Read the model definition and answer for the solid it produces. Units are mm, in the model's axes. A direction names the side the tool comes from. Coordinates: 2 decimals unless noted, no trailing zeros. Write each loop counter-clockwise with the first axis right and the second up, starting at its lowest first coordinate (ties: lowest second). Pieces come first, ordered by that corner, then holes.
1) Determine the mould class of faces 5 (the face through (10, 8, 0)), 6 (the face through (18.44, -17.48, 9.1)), 7 (the face through (-13.64, -17.48, -0.37)), 8 (the face through (0, -19, 0)) for opening direction Z: +Z half, -Z half, draft (parallel to the pull), parting line (faces both ways), or undercut.
2) The part is cut by section D-D (x = 0). Determine the outline of the cut face in (y, z), then the cut area to 3 significant figures.
3) Which of the six approach directions +Z, -Z, +X, -X, +Y, -Y give full straight-line access (tool end or side, diameter ignored) to faces 1 (the face through (10, -1, -8)), 2 (the face through (13, -16, 0)), 3 (the face through (7.9, -10, 9)), 4 (the face through (0, -6, -8))?
4) Find the intervals of material crossed by line 1 (X direction, y = -16.95, z = 0); line 2 (Z direction, x = 0, y = -16.8); line 3 (X direction, y = -9.5, z = -3), in increasing order.
5) Each of these flat-tipped pins is pushed along its axis until it touches: pin 1 Ø5.5 at (x, z) = (15.3, 0) entering from +Y; pin 2 Ø5 at (x, y) = (-9.5, 1) entering from -Z; pin 3 Ø3 at (x, z) = (0, 7.5) entering from +Y; pin 4 Ø3 at (y, z) = (-12, -5.318) entering from +X. Where does it stop, or does it pass through?
6) The part is cut by section C-C (y = -15). Determine the outline of the cut face in (x, z).
7) The part is cut by section A-A (x = -15.3). Determine the outline of the cut face in (y, z), then the cut area to 3 significant figures.
8) The part is cut by section B-B (z = 0). Determine the outline of the cut face in (x, y).
from build123d import *

# Parameters (mm, degrees)
ESQUISSE2_W                    = 2.5
ESQUISSE2_H                    = 6
BOSS_EXTRU_1_START             = -2.5
ESQUISSE3_R                    = 2
BOSS_EXTRU_1_DEPTH             = 2.5
BOSS_EXTRU_2_START             = -2.5
ESQUISSE3_3_W                  = 20
ESQUISSE3_3_H                  = 3
ESQUISSE3_3_W_2                = 2
BOSS_EXTRU_2_DEPTH             = 8.8
ESQUISSE3_5_W                  = 20
ESQUISSE3_5_H                  = 3
BOSS_EXTRUDE1_DEPTH            = 8
CUT_EXTRUDE1_REACH             = 34.38
SKETCH4_R                      = 1.7
TROUS_DE_CENTRAGE_2_0MM1_D     = 2
TROUS_DE_CENTRAGE_2_0MM1_DEPTH = 3
FILLET1_R                      = 1
FILLET2_START                  = -8.8
FILLET2_DEPTH                  = 17.6
FILLET2_START_2                = -19.3
FILLET2_2_DEPTH                = 38.6
FILLET3_R                      = 3


with BuildPart() as part:
    # Esquisse2 → Révolution1 (revolve)
    with BuildSketch(Plane.XY, mode=Mode.PRIVATE) as r_volution1_sk:
        with Locations((10.05, 5)):
            Rectangle(ESQUISSE2_W, ESQUISSE2_H)
    revolve(r_volution1_sk.sketch.rotate(Axis((-2.14668318, 0, 0), (1, 0, 0)), 90), axis=Axis((-2.14668318, 0, 0), (1, 0, 0)))

    # Esquisse3 → Boss.-Extru.1 (add)
    with BuildSketch(Plane(origin=(11.3, 0, 0), x_dir=(0, 0, -1), z_dir=(1, 0, 0)).offset(BOSS_EXTRU_1_START)):
        with BuildLine():
            Line((-10, -19), (10, -19))
            Line((10, -19), (10, -3.313708499))
            Line((10, -3.313708499), (8, -3.313708499))
            Line((8, -3.313708499), (8, 0))
            ThreePointArc((8, 0), (0, -8), (-8, 0))
            Line((-8, 0), (-8, -6.142135624))
            Line((-8, -6.142135624), (-10, -6.142135624))
            Line((-10, -6.142135624), (-10, -19))
        make_face()
        with Locations((5.318, -12)):
            Circle(ESQUISSE3_R, mode=Mode.SUBTRACT)
    extrude(amount=BOSS_EXTRU_1_DEPTH)

    # Esquisse3<3> → Boss.-Extru.2 (add)
    with BuildSketch(Plane(origin=(11.3, 0, 0), x_dir=(0, 0, -1), z_dir=(1, 0, 0)).offset(BOSS_EXTRU_2_START)):
        with Locations((0, -17.5)):
            Rectangle(ESQUISSE3_3_W, ESQUISSE3_3_H)
        with Locations((-9, -7.642135624)):
            Rectangle(ESQUISSE3_3_W_2, ESQUISSE3_3_H)
        with Locations((9, -4.813708499)):
            Rectangle(ESQUISSE3_3_W_2, ESQUISSE3_3_H)
    extrude(amount=-BOSS_EXTRU_2_DEPTH)

    # Esquisse3<5> → Boss-Extrude1 (add)
    with BuildSketch(Plane(origin=(11.3, 0, 0), x_dir=(0, 0, -1), z_dir=(1, 0, 0))):
        with Locations((0, -17.5)):
            Rectangle(ESQUISSE3_5_W, ESQUISSE3_5_H)
    extrude(amount=BOSS_EXTRUDE1_DEPTH)

    # Sketch4 → Cut-Extrude1 (cut, up to next)
    with BuildSketch(Plane(origin=(0, -16, 0), x_dir=(1, 0, 0), z_dir=(0, 1, 0)), mode=Mode.PRIVATE) as cut_extrude1_sk1:
        with Locations(Location((15.3, 0, 0), (0, 0, 270))):
            Circle(SKETCH4_R)
    cut_extrude1_tool1 = extrude(cut_extrude1_sk1.sketch, amount=-CUT_EXTRUDE1_REACH, mode=Mode.PRIVATE) & part.part
    add(cut_extrude1_tool1.solids().sort_by_distance((15.3, -16, 0))[0], mode=Mode.SUBTRACT)

    # Symétrie1: part across plane


with BuildPart() as part_1:
    add(part.part)
    add(part.part.mirror(Plane(origin=(0, 0, 0), x_dir=(0, 0, 1), z_dir=(1, 0, 0))))

    # Trous de centrage Ø2.0mm1
    with Locations(Plane(origin=(0, -16, 0), x_dir=(1, 0, 0), z_dir=(0, 1, 0))):
        with Locations((0, -7.5)):
            Hole(TROUS_DE_CENTRAGE_2_0MM1_D / 2, depth=TROUS_DE_CENTRAGE_2_0MM1_DEPTH)

    # Fillet1
    fillet1_edges = [part_1.edges().sort_by_distance(p)[0] for p in [
        (-10.05, -3.313708499, -8),
        (-10.05, -6.142135624, 8),
        (10.05, -3.313708499, -8),
        (10.05, -6.142135624, 8),
    ]]
    fillet(fillet1_edges, radius=FILLET1_R)

    # Fillet2: read off the stored shape, not the designer's step
    # Fillet2 outline → Fillet2 (cut)
    with BuildSketch(Plane.YZ.offset(FILLET2_START)):
        with BuildLine():
            ThreePointArc((-4.313708499, -8), (-3.606601718, -8.292893219), (-3.313708499, -9))
            Line((-3.313708499, -9), (-3.313708499, -8))
            Line((-3.313708499, -8), (-4.313708499, -8))
        make_face()
        with BuildLine():
            ThreePointArc((-3.313708499, -9), (-3.606601718, -9.707106781), (-4.313708499, -10))
            Line((-4.313708499, -10), (-3.313708499, -10))
            Line((-3.313708499, -10), (-3.313708499, -9))
        make_face()
        with BuildLine():
            Line((-6.142135624, 8), (-6.142135624, 9))
            ThreePointArc((-6.142135624, 9), (-6.435028843, 8.292893219), (-7.142135624, 8))
            Line((-7.142135624, 8), (-6.142135624, 8))
        make_face()
        with BuildLine():
            ThreePointArc((-7.142135624, 10), (-6.435028843, 9.707106781), (-6.142135624, 9))
            Line((-6.142135624, 9), (-6.142135624, 10))
            Line((-6.142135624, 10), (-7.142135624, 10))
        make_face()
    extrude(amount=FILLET2_DEPTH, mode=Mode.SUBTRACT)

    # Fillet2 2 outline → Fillet2 2 (cut)
    with BuildSketch(Plane.YZ.offset(FILLET2_START_2)):
        with BuildLine():
            ThreePointArc((-3.313708499, -9), (-3.606601718, -9.707106781), (-4.313708499, -10))
            Line((-4.313708499, -10), (-3.313708499, -10))
            Line((-3.313708499, -10), (-3.313708499, -9))
        make_face()
        with BuildLine():
            ThreePointArc((-7.142135624, 10), (-6.435028843, 9.707106781), (-6.142135624, 9))
            Line((-6.142135624, 9), (-6.142135624, 10))
            Line((-6.142135624, 10), (-7.142135624, 10))
        make_face()
    extrude(amount=FILLET2_2_DEPTH, mode=Mode.SUBTRACT)

    # Fillet3
    fillet3_edges = [part_1.edges().sort_by_distance(p)[0] for p in [
        (-8.8, -6.313708499, -9),
        (-19.3, -17.5, -10),
        (8.8, -6.313708499, -9),
        (8.8, -9.142135624, 9),
        (19.3, -17.5, -10),
        (19.3, -17.5, 10),
        (-8.8, -9.142135624, 9),
        (-19.3, -17.5, 10),
    ]]
    fillet(fillet3_edges, radius=FILLET3_R)


solid = part_1.part
Reported:
1. face 5: parting line
1. face 6: +Z half
1. face 7: undercut
1. face 8: draft
2. outline: (-19, -10) - (-16, -10) - (-16, 6.5) - (-19, 6.5) - close; (-19, 8.5) - (-16, 8.5) - (-16, 10) - (-19, 10) - close; (-9.14, 8) - (-7.14, 8) arc R1 ccw to (-7.14, 10) - (-9.14, 10) - close; (-6.31, -10) - (-4.31, -10) arc R1 ccw to (-4.31, -8) - (-6.31, -8) - close
2. area: 65.1 mm2
3. face 1: -Z, +X, -X, +Y
3. face 2: +Z, -Z, +X, +Y
3. face 3: +Z, -Z
3. face 4: +Y
4. line 1: x = -19.3 to -17, -13.6 to 13.6, 17 to 19.3
4. line 2: z = -10 to 6.5, 8.5 to 10
4. line 3: x = -11.3 to -8.8, 8.8 to 11.3
5. pin 1: stops at y = -16
5. pin 2: stops at z = -8
5. pin 3: stops at y = -6.14
5. pin 4: passes through
6. outline: (-11.3, -10) - (-8.8, -10) - (-8.8, 10) - (-11.3, 10) - close; (8.8, -10) - (11.3, -10) - (11.3, 10) - (8.8, 10) - close
7. outline: (-19, -10) - (-16, -10) - (-16, -1.7) - (-19, -1.7) - close; (-19, 1.7) - (-16, 1.7) - (-16, 10) - (-19, 10) - close
7. area: 49.8 mm2
8. outline: (-19.3, -19) - (-17, -19) - (-17, -16) - (-19.3, -16) - close; (-13.6, -19) - (13.6, -19) - (13.6, -16) - (11.3, -16) - (11.3, -2) - (8.8, -2) - (8.8, -16) - (-8.8, -16) - (-8.8, -2) - (-11.3, -2) - (-11.3, -16) - (-13.6, -16) - close; (-11.3, 2) - (-8.8, 2) - (-8.8, 8) - (-11.3, 8) - close; (8.8, 2) - (11.3, 2) - (11.3, 8) - (8.8, 8) - close; (17, -19) - (19.3, -19) - (19.3, -16) - (17, -16) - close
